Geometry check sheet. Reference: the model listing, model coordinates, mm. Face numbers are marked on the shaded views. Give positions to 0.01 mm unless a question says otherwise; leave off trailing zeros. Loops run counter-clockwise (first coordinate to the right, second up) from the corner with the lowest first, then second, coordinate; pieces in that order, holes last.
1. Go/stop test with flat-tipped pins: pin 1 Ø3 at (x, z) = (-13.5, -32.5) entering from -Y; pin 2 Ø1.8 at (x, z) = (8.5, -43.5) entering from +Y; pin 3 Ø5 at (y, z) = (8.5, 15.5) entering from +X; pin 4 Ø4 at (x, y) = (-14.5, 5.5) entering from +Z. Record where each tip stops, or that it passes through.
2. Cross-section at C-C, the plane y = 5.5. State how many separate pieces and enclosed holes the cut face has, plus the area to 3 significant figures.
3. Release check for a two-part mould opening along X. For the marked faces 1, 2 and 3 record: +X half, -X half, draft (parallel to the pull), parting line (faces both ways), or undercut.
4. Cross-section at A-A, the plane z = 0. Record the cut outline in (x, y), plus the area to 3 significant figures.
5. Cross-section at B-B, the plane x = -19.5. Record the cut outline in (y, z), plus the area to 3 significant figures.
6. Cross-section at D-D, the plane x = -1.5. Record the cut outline in (y, z).
7. Material ranges on L1, parallel to X at y = 4.75, z = 0.5; L2, parallel to Z at x = 25, y = 12.25; L3, parallel to X at y = 11, z = 7, recorded low to high.
from build123d import *

# Parameters (mm, degrees)
SKETCH1_R           = 50
SKETCH1_R_2         = 24
BOSS_EXTRUDE1_DEPTH = 13.2
SKETCH2_R           = 2
CUT_EXTRUDE3_DEPTH  = 13.2
SKETCH2_6_R         = 3
CUT_EXTRUDE4_DEPTH  = 2
CIRPATTERN2_COUNT   = 8
CIRPATTERN3_COUNT   = 8
SKETCH3_R           = 2.75
CUT_EXTRUDE5_DEPTH  = 4.2
CIRPATTERN4_COUNT   = 16
CUT_EXTRUDE9_START  = -9.2
SKETCH5_R           = 27.5
SKETCH5_R_2         = 24
CUT_EXTRUDE9_DEPTH  = 9.2


with BuildPart() as part:
    # Sketch1 → Boss-Extrude1 (new body)
    with BuildSketch(Plane(origin=(0, 0, 0), x_dir=(1, 0, 0), z_dir=(0, 1, 0))):
        with Locations(Location((0, 0, 0), (0, 0, 270))):
            Circle(SKETCH1_R)
        with Locations(Location((0, 0, 0), (0, 0, 270))):
            Circle(SKETCH1_R_2, mode=Mode.SUBTRACT)
    extrude(amount=BOSS_EXTRUDE1_DEPTH)

    # Sketch2 → Cut-Extrude3 (cut)
    with BuildSketch(Plane(origin=(0, 13.2, 0), x_dir=(1, 0, 0), z_dir=(0, 1, 0))):
        with Locations(Location((37.416132554, 25.000660486, 0), (0, 0, 270))):
            Circle(SKETCH2_R)
    cut_extrude3 = extrude(amount=-CUT_EXTRUDE3_DEPTH, mode=Mode.SUBTRACT)

    # Sketch2_6 → Cut-Extrude4 (cut)
    with BuildSketch(Plane(origin=(0, 13.2, 0), x_dir=(1, 0, 0), z_dir=(0, 1, 0))):
        with Locations(Location((37.416132554, 25.000660486, 0), (0, 0, 270))):
            Circle(SKETCH2_6_R)
    cut_extrude4 = extrude(amount=-CUT_EXTRUDE4_DEPTH, mode=Mode.SUBTRACT)

    # CirPattern2: Cut-Extrude3 ×8 about axis
    cirpattern2_axis = Axis((0, 0, 0), (0, 1, 0))
    for i in range(1, CIRPATTERN2_COUNT):
        add(cut_extrude3.rotate(cirpattern2_axis, i * 360 / CIRPATTERN2_COUNT), mode=Mode.SUBTRACT)

    # CirPattern3: Cut-Extrude4 ×8 about axis
    cirpattern3_axis = Axis((0, 0, 0), (0, 1, 0))
    for i in range(1, CIRPATTERN3_COUNT):
        add(cut_extrude4.rotate(cirpattern3_axis, i * 360 / CIRPATTERN3_COUNT), mode=Mode.SUBTRACT)

    # Sketch3 → Cut-Extrude5 (cut)
    with BuildSketch(Plane.XZ):
        with Locations(Location((0, 35, 0), (0, 0, 270))):
            Circle(SKETCH3_R)
    cut_extrude5 = extrude(amount=-CUT_EXTRUDE5_DEPTH, mode=Mode.SUBTRACT)

    # CirPattern4: Cut-Extrude5 ×16 about axis
    cirpattern4_axis = Axis((0, 0, 0), (0, 1, 0))
    for i in range(1, CIRPATTERN4_COUNT):
        add(cut_extrude5.rotate(cirpattern4_axis, i * 360 / CIRPATTERN4_COUNT), mode=Mode.SUBTRACT)

    # Sketch5 → Cut-Extrude9 (cut)
    with BuildSketch(Plane(origin=(0, 13.2, 0), x_dir=(1, 0, 0), z_dir=(0, 1, 0)).offset(CUT_EXTRUDE9_START)):
        with Locations(Location((0, 0, 0), (0, 0, 270))):
            Circle(SKETCH5_R)
        with Locations(Location((0, 0, 0), (0, 0, 270))):
            Circle(SKETCH5_R_2, mode=Mode.SUBTRACT)
    extrude(amount=CUT_EXTRUDE9_DEPTH, mode=Mode.SUBTRACT)


solid = part.part
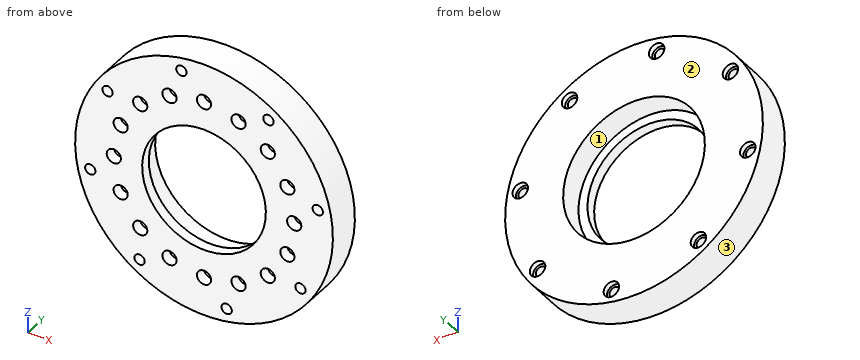
Result:
1. pin 1: stops at y = 4.2
1. pin 2: passes through
1. pin 3: stops at x = 48.28
1. pin 4: stops at z = 48.41
2. separate pieces: 1
2. enclosed holes: 9
2. area: 5,380 mm2
3. face 1: undercut
3. face 2: draft
3. face 3: parting line
4. outline: (-50, 0) - (-37.75, 0) - (-37.75, 4.2) - (-32.25, 4.2) - (-32.25, 0) - (-24, 0) - (-24, 4) - (-27.5, 4) - (-27.5, 13.2) - (-50, 13.2) - close; (24, 0) - (32.25, 0) - (32.25, 4.2) - (37.75, 4.2) - (37.75, 0) - (50, 0) - (50, 13.2) - (27.5, 13.2) - (27.5, 4) - (24, 4) - close
4. area: 576 mm2
5. outline: (0, -46.04) - (13.2, -46.04) - (13.2, -19.39) - (4, -19.39) - (4, -13.99) - (0, -13.99) - close; (0, 13.99) - (4, 13.99) - (4, 19.39) - (13.2, 19.39) - (13.2, 46.04) - (0, 46.04) - close
5. area: 747 mm2
6. outline: (0, -49.98) - (13.2, -49.98) - (13.2, -27.46) - (4, -27.46) - (4, -23.95) - (0, -23.95) - (0, -32.7) - (4.2, -32.7) - (4.2, -37.3) - (0, -37.3) - close; (0, 23.95) - (4, 23.95) - (4, 27.46) - (13.2, 27.46) - (13.2, 49.98) - (0, 49.98) - (0, 37.3) - (4.2, 37.3) - (4.2, 32.7) - (0, 32.7) - close
7. L1: x = -50 to -27.5, 27.5 to 50
7. L2: z = -43.3 to -11.46, 11.46 to 34.42, 40.42 to 43.3
7. L3: x = -49.51 to -26.59, 26.59 to 43.22, 45.05 to 49.51
